from build123d import *

# Parameters (mm, degrees)
SKETCH1_R           = 7.9375
BOSS_EXTRUDE1_DEPTH = 4.7625
SKETCH2_R           = 6.35
BOSS_EXTRUDE2_DEPTH = 10.16
SKETCH3_R           = 2.7051
CUT_EXTRUDE1_DEPTH  = 19.67321126


with BuildPart() as part:
    # Sketch1 → Boss-Extrude1 (new body)
    with BuildSketch(Plane(origin=(0, 0, 0), x_dir=(1, 0, 0), z_dir=(0, 1, 0))):
        with Locations(Location((0, 0, 0), (0, 0, 90))):
            Circle(SKETCH1_R)
    extrude(amount=BOSS_EXTRUDE1_DEPTH)

    # Sketch2 → Boss-Extrude2 (add)
    with BuildSketch(Plane(origin=(0, 4.7625, 0), x_dir=(1, 0, 0), z_dir=(0, 1, 0))):
        with Locations(Location((0, 0, 0), (0, 0, 270))):
            Circle(SKETCH2_R)
    extrude(amount=BOSS_EXTRUDE2_DEPTH)

    # Sketch3 → Cut-Extrude1 (cut, through all)
    with BuildSketch(Plane(origin=(0, 14.9225, 0), x_dir=(1, 0, 0), z_dir=(0, 1, 0))):
        with Locations(Location((0, 0, 0), (0, 0, 270))):
            Circle(SKETCH3_R)
    extrude(amount=-CUT_EXTRUDE1_DEPTH, mode=Mode.SUBTRACT)


solid = part.part
Part model, mm, in its own coordinate system. A direction names the side the tool comes from. Round coordinates to 2 decimals unless told otherwise and drop trailing zeros. Write each loop counter-clockwise with the first axis right and the second up, starting at its lowest first coordinate (ties: lowest second). Pieces come first, ordered by that corner, then holes. Notation, with made-up numbers: M 27.25,13.25 L 69.25,13.25 A16 ccw 69.25,39.25 Z; hole C 19,11 d1. An arc over 180 degrees is marked long. Return JSON: item names as keys, results as strings. Group by question number.
(1) Drill centre lines: probe 1 along X at (y, z) = (4, 0); probe 2 along X at (y, z) = (6.5, 0); probe 3 along Z at (x, y) = (1.5, 13). Where is each one in solid material? Low to high.
(2) Two-plate mould, pull along Z, no slides. Class faces 3 (the face through (0, 14.922, 3)), 4 (the face through (0.81, 7.57, 2.58)), 5 (the face through (7.75, 2.35, 1.72)): +Z half, -Z half, draft (parallel to the pull), parting line (faces both ways), or undercut.
(3) Saw through at A-A on x = 0. Write the cut outline in (y, z).
(4) Saw through at D-D on z = -3.25. Write the cut outline in (x, y), then the cut area to 3 significant figures.
(5) Which spindle directions (+Z, -Z, +X, -X, +Y, -Y) get a long thin tool onto all of the face, cutting with end or side? Do faces 1 (the face through (3, 0, 0)), 2 (the face through (-3.86, 9.77, -5.04)). Say none if no direction does.
(6) Pin check, flat tips, straight feed: pin 1 Ø4 at (y, z) = (4.5, 5.5) entering from +X; pin 2 Ø4 at (y, z) = (7, -6) entering from -X. Stop position of each tip, or through.
(7) Saw through at C-C on y = 8.75. Write the cut outline in (x, z).
(8) Saw through at B-B on z = 0. Write the cut outline in (x, y), then the cut area to 3 significant figures.
Returned:
{
 "1": {"probe 1": "-7.94 to -2.71, 2.71 to 7.94", "probe 2": "-6.35 to -2.71, 2.71 to 6.35", "probe 3": "-6.17 to -2.25, 2.25 to 6.17"},
 "2": {"face 3": "draft", "face 4": "undercut", "face 5": "parting line"},
 "3": {"outline": "M 0,-7.94 L 4.76,-7.94 L 4.76,-6.35 L 14.92,-6.35 L 14.92,-2.71 L 0,-2.71 Z; M 0,2.71 L 14.92,2.71 L 14.92,6.35 L 4.76,6.35 L 4.76,7.94 L 0,7.94 Z"},
 "4": {"outline": "M -7.24,0 L 7.24,0 L 7.24,4.76 L 5.46,4.76 L 5.46,14.92 L -5.46,14.92 L -5.46,4.76 L -7.24,4.76 Z", "area": "180 mm²"},
 "5": {"face 1": "+Z, -Z, +X, -X, -Y", "face 2": "+Y"},
 "6": {"pin 1": "x = 7.12", "pin 2": "x = -4.93"},
 "7": {"outline": "C 0,0 d12.7; hole C 0,0 d5.41"},
 "8": {"outline": "M -7.94,0 L -2.71,0 L -2.71,14.92 L -6.35,14.92 L -6.35,4.76 L -7.94,4.76 Z; M 2.71,0 L 7.94,0 L 7.94,4.76 L 6.35,4.76 L 6.35,14.92 L 2.71,14.92 Z", "area": "124 mm²"}
}
